Geometry check sheet. Reference: the model listing, model coordinates, mm. A direction names the side the tool comes from. Give positions to 0.01 mm unless a question says otherwise; leave off trailing zeros. Write each loop counter-clockwise with the first axis right and the second up, starting at its lowest first coordinate (ties: lowest second). Pieces come first, ordered by that corner, then holes. Notation, with made-up numbers: (-35.5, -29) -> (7.5, -29) arc R34 ccw to (7.5, 10) -> close; hole circle Ø5 at (15.5, 66). An arc over 180 degrees is marked (long way). Use a Markdown table: item, result. Add a question column.
from build123d import *

# Parameters (mm, degrees)
SKETCH1_W                     = 37
SKETCH1_H                     = 45
BOSS_EXTRUDE1_DEPTH           = 1
BOSS_EXTRUDE2_DEPTH           = 1
FILLET1_R                     = 3
M3_CLEARANCE_HOLE1_AT_2_COUNT = 2
M3_CLEARANCE_HOLE1_AT_2_PITCH = 37
M3_CLEARANCE_HOLE1_AT_3_COUNT = 2
M3_CLEARANCE_HOLE1_AT_3_PITCH = 56.727418415
M3_CLEARANCE_HOLE1_AT_4_COUNT = 2
M3_CLEARANCE_HOLE1_AT_4_PITCH = 43


with BuildPart() as part:
    # Sketch1 → Boss-Extrude1 (new body)
    with BuildSketch(Plane(origin=(0, 0, 0), x_dir=(1, 0, 0), z_dir=(0, 1, 0))):
        Rectangle(SKETCH1_W, SKETCH1_H)
    extrude(amount=BOSS_EXTRUDE1_DEPTH)

    # Sketch2 → Boss-Extrude2 (add)
    with BuildSketch(Plane.XZ):
        with BuildLine():
            Line((21.5, 14.5), (-21.5, 14.5))
            ThreePointArc((-21.5, 14.5), (-25.5, 18.5), (-21.5, 22.5))
            Line((-21.5, 22.5), (21.5, 22.5))
            ThreePointArc((21.5, 22.5), (25.5, 18.5), (21.5, 14.5))
        make_face()
        with BuildLine():
            Line((21.5, -14.5), (-21.5, -14.5))
            ThreePointArc((-21.5, -14.5), (-25.5, -18.5), (-21.5, -22.5))
            Line((-21.5, -22.5), (21.5, -22.5))
            ThreePointArc((21.5, -22.5), (25.5, -18.5), (21.5, -14.5))
        make_face()
    extrude(amount=-BOSS_EXTRUDE2_DEPTH)

    # Fillet1
    fillet1_edges = [part.edges().sort_by_distance(p)[0] for p in [
        (-18.5, 0.5, 14.5),
        (-18.5, 0.5, -14.5),
        (18.5, 0.5, -14.5),
        (18.5, 0.5, 14.5),
    ]]
    fillet(fillet1_edges, radius=FILLET1_R - 0.0001)  # a hair under: the kernel refuses the full size

    # Sketch5 → M3 Clearance Hole1 (revolve, cut)
    with BuildSketch(Plane(origin=(-21.5, 1, -18.5), x_dir=(0, 0, 1), z_dir=(1, 0, 0))):
        Polygon((0, 0), (0, 1), (1.7, 1), (1.7, 0.025), (1.725, 0), align=None)
    m3_clearance_hole1 = revolve(axis=Axis((-21.5, 7.35, -18.5), (0, -1, 0)), mode=Mode.SUBTRACT)

    # M3 Clearance Hole1 at 2: M3 Clearance Hole1 ×2
    with Locations(*[(0, 0, i * M3_CLEARANCE_HOLE1_AT_2_PITCH) for i in range(1, M3_CLEARANCE_HOLE1_AT_2_COUNT)]):
        add(m3_clearance_hole1, mode=Mode.SUBTRACT)

    # M3 Clearance Hole1 at 3: M3 Clearance Hole1 ×2
    with Locations(*[Vector(0.7580108737829233, 0, 0.6522419146504225) * (i * M3_CLEARANCE_HOLE1_AT_3_PITCH) for i in range(1, M3_CLEARANCE_HOLE1_AT_3_COUNT)]):
        add(m3_clearance_hole1, mode=Mode.SUBTRACT)

    # M3 Clearance Hole1 at 4: M3 Clearance Hole1 ×2
    with Locations(*[(i * M3_CLEARANCE_HOLE1_AT_4_PITCH, 0, 0) for i in range(1, M3_CLEARANCE_HOLE1_AT_4_COUNT)]):
        add(m3_clearance_hole1, mode=Mode.SUBTRACT)


solid = part.part
1) Tool access check on faces 5 (the face through (19.4, 0.51, 13.64)), 6 (the face through (23, 0.5, 19.3)), 7 (the face through (-19.4, 0.51, 13.64)). Record the directions out of +Z, -Z, +X, -X, +Y, -Y that give a thin tool (end or side, any length) a straight path to the whole face; none if there is none.
2) Sectioned sample at A-A, the plane z = -18.5. Enter the section's corners in (x, y) (3 decimals).
3) Gauge pin test, flat end, axial feed: P1, Ø0.5, axis at y = 0.5, z = -2.5, coming from the -X side. Record the tip position at first contact, or that the pin passes through.
4) Sectioned sample at C-C, the plane z = -5. Enter the section's corners in (x, y).
5) Draft check along X on faces 1 (the face through (-22.01, 0.49, -16.88)), 2 (the face through (-19.36, 0.51, -13.6)), 3 (the face through (0, 1, 0)), 4 (the face through (19.4, 0.51, -13.64)). Enter one of: +X half, -X half, draft (parallel to the pull), parting line (faces both ways), or undercut.
6) Sectioned sample at B-B, the plane y = 0.15. Count the separate pieces of the cut face and the enclosed holes in it, and give its area (3 significant figures).
7) Material ranges on probe 1 along X at (y, z) = (0.75, 18.5); probe 2 along Z at (x, y) = (-21.5, 0.5); probe 3 along X at (y, z) = (0.35, 18), recorded low to high. Write a range as [from, to].
Check values:
| question | item | result |
|---|---|---|
| 1 | face 5 | +X, +Y, -Y |
| 1 | face 6 | +Y, -Y |
| 1 | face 7 | -X, +Y, -Y |
| 2 | outline | (-25.5, 0) -> (-23.2, 0) -> (-23.2, 0.975) -> (-23.225, 1) -> (-25.5, 1) -> close; (-19.8, 0) -> (19.8, 0) -> (19.8, 0.975) -> (19.775, 1) -> (-19.775, 1) -> (-19.8, 0.975) -> close; (23.2, 0) -> (25.5, 0) -> (25.5, 1) -> (23.225, 1) -> (23.2, 0.975) -> close |
| 3 | P1 | x = -18.5 |
| 4 | outline | (-18.5, 0) -> (18.5, 0) -> (18.5, 1) -> (-18.5, 1) -> close |
| 5 | face 1 | undercut |
| 5 | face 2 | -X half |
| 5 | face 3 | draft |
| 5 | face 4 | +X half |
| 6 | separate pieces | 1 |
| 6 | enclosed holes | 4 |
| 6 | area | 1,830 mm² |
| 7 | probe 1 | [-25.5, -23.2], [-19.8, 19.8], [23.2, 25.5] |
| 7 | probe 2 | [-22.5, -20.2], [-16.8, -14.5], [14.5, 16.8], [20.2, 22.5] |
| 7 | probe 3 | [-25.47, -23.12], [-19.88, 19.88], [23.12, 25.47] |
